Work out the finished part from the listing and answer in its coordinate system (mm). Face numbers are marked on the shaded views. Coordinates: 2 decimals unless noted, no trailing zeros. Loops run counter-clockwise (first coordinate to the right, second up) from the corner with the lowest first, then second, coordinate; pieces in that order, holes last. Notation, with made-up numbers: (21, -17) -> (37, -17) arc R25 cw to (37, -1) -> close; hole circle Ø1 at (74.25, 80.25). An arc over 180 degrees is marked (long way). Use a Markdown table: item, result. Add a question column.
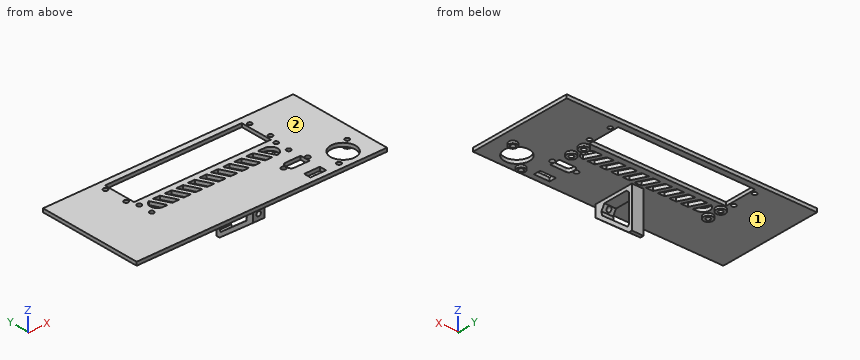
```python
from build123d import *
from OCP.BRepFilletAPI import BRepFilletAPI_MakeChamfer

# Parameters (mm, degrees)
SZKIC1_W                    = 215
SZKIC1_H                    = 90
DODANIE_WYCI_GNI_CIE1_DEPTH = 3
DODANIE_WYCI_GNI_CIE3_DEPTH = 5
SZKIC4_R                    = 1.9
WYTNIJ_WYCI_GNI_CIE1_DEPTH  = 10
SZKIC5_R                    = 1.9
SZKIC5_W                    = 117.5
SZKIC5_H                    = 28
WYTNIJ_WYCI_GNI_CIE2_DEPTH  = 35
SFAZOWANIE1_SIZE            = 2
SFAZOWANIE1_SIZE2           = 1.42483793
SFAZOWANIE1_SIZE2_2         = 2.349845037
SZKIC6_R                    = 10.75
SZKIC6_R_2                  = 1.9
SZKIC6_R_3                  = 2
SZKIC6_W                    = 13.5
SZKIC6_H                    = 6
WYTNIJ_WYCI_GNI_CIE3_DEPTH  = 237.154610372
SZKIC8_R                    = 3.5
SZKIC8_R_2                  = 2
DODANIE_WYCI_GNI_CIE4_DEPTH = 2
SZKIC9_R                    = 1.9
WYTNIJ_WYCI_GNI_CIE4_DEPTH  = 3
DODANIE_WYCI_GNI_CIE5_START = 2
SZKIC10_R                   = 4
SZKIC10_R_2                 = 1.9
DODANIE_WYCI_GNI_CIE5_DEPTH = 2


with BuildPart() as part:
    # Szkic1 → Dodanie-wyciągnięcie1 (new body)
    with BuildSketch(Plane.XY):
        with Locations((107.5, 45)):
            Rectangle(SZKIC1_W, SZKIC1_H)
    extrude(amount=DODANIE_WYCI_GNI_CIE1_DEPTH)

    # Szkic3 → Dodanie-wyciągnięcie3 (add, symmetric)
    with BuildSketch(Plane(origin=(107.5, 0, 0), x_dir=(0, 0, -1), z_dir=(1, 0, 0))):
        Polygon((0, 3), (10, 3), (35, 35), (35, 38), (0, 38), align=None)
        Polygon((3, 11.541451884), (3, 35), (31.193011155, 35), (9.799205499, 7.615928759), align=None, mode=Mode.SUBTRACT)
    extrude(amount=DODANIE_WYCI_GNI_CIE3_DEPTH, both=True)

    # Szkic4 → Wytnij-wyciągnięcie1 (cut)
    with BuildSketch(Plane.XZ.offset(-3)):
        with Locations(Location((107.5, -5, 0), (0, 0, 270))):
            Circle(SZKIC4_R)
    extrude(amount=-WYTNIJ_WYCI_GNI_CIE1_DEPTH, mode=Mode.SUBTRACT)

    # Szkic5 → Wytnij-wyciągnięcie2 (cut)
    with BuildSketch(Plane.XY.offset(3)):
        with Locations((45.5, 81)):
            Circle(SZKIC5_R)
        with Locations((45.5, 61)):
            Circle(SZKIC5_R)
        with Locations((169.5, 61)):
            Circle(SZKIC5_R)
        with Locations((169.5, 81)):
            Circle(SZKIC5_R)
        with Locations((107.5, 71)):
            Rectangle(SZKIC5_W, SZKIC5_H)
    extrude(amount=-WYTNIJ_WYCI_GNI_CIE2_DEPTH, mode=Mode.SUBTRACT)

    # Sfazowanie1: one chamfer whose edges measure the first distance from different faces: ONE call of the kernel's chamfer builder (chamfer() names one face for all edges)
    sfazowanie1_edges_1 = [part.edges().sort_by_distance(p)[0] for p in [
        (107.5, 35, -31.193011155),
    ]]
    sfazowanie1_side_1 = [part.faces().sort_by_distance(p)[0] for p in [
        (107.5, 35, -17.096505578),
    ]]
    sfazowanie1_edges_2 = [part.edges().sort_by_distance(p)[0] for p in [
        (107.5, 35, -3),
    ]]
    sfazowanie1_edges_3 = [part.edges().sort_by_distance(p)[0] for p in [
        (107.5, 7.615928759, -9.799205499),
    ]]
    sfazowanie1_side_3 = [part.faces().sort_by_distance(p)[0] for p in [
        (107.5, 21.30796438, -20.496108327),
    ]]
    sfazowanie1 = BRepFilletAPI_MakeChamfer(part.part.solid().wrapped)
    for e in sfazowanie1_edges_1:
        sfazowanie1.Add(SFAZOWANIE1_SIZE, SFAZOWANIE1_SIZE2, e.wrapped, sfazowanie1_side_1[0].wrapped)  # the first distance lies on this face
    for e in sfazowanie1_edges_2:
        sfazowanie1.Add(SFAZOWANIE1_SIZE, e.wrapped)
    for e in sfazowanie1_edges_3:
        sfazowanie1.Add(SFAZOWANIE1_SIZE, SFAZOWANIE1_SIZE2_2, e.wrapped, sfazowanie1_side_3[0].wrapped)  # the first distance lies on this face
    add(Compound.cast(sfazowanie1.Shape()), mode=Mode.REPLACE)

    # Szkic6 → Wytnij-wyciągnięcie3 (cut, through all)
    with BuildSketch(Plane.XY.offset(3)):
        with Locations((191, 15.35)):
            Circle(SZKIC6_R)
        with Locations((203, 24.85)):
            Circle(SZKIC6_R_2)
        with Locations((179, 5.85)):
            Circle(SZKIC6_R_2)
        with Locations((148.5, 25.05)):
            Circle(SZKIC6_R_3)
        with Locations((169.25, 25.05)):
            Circle(SZKIC6_R_3)
        with Locations((160.25, 7.8)):
            Rectangle(SZKIC6_W, SZKIC6_H)
        with BuildLine():
            Line((167, 20.8), (153.9, 20.8))
            ThreePointArc((153.9, 20.8), (151.849390335, 21.649390335), (151, 23.7))
            Line((151, 23.7), (151, 26.4))
            ThreePointArc((151, 26.4), (151.849390335, 28.450609665), (153.9, 29.3))
            Line((153.9, 29.3), (167, 29.3))
            Line((167, 29.3), (167, 20.8))
        make_face()
    extrude(amount=-WYTNIJ_WYCI_GNI_CIE3_DEPTH, mode=Mode.SUBTRACT)

    # Szkic8 → Dodanie-wyciągnięcie4 (add)
    # profile 1 of 2: a face of its own
    with BuildSketch(Plane(origin=(0, 0, 0), x_dir=(-1, 0, 0), z_dir=(0, 0, -1))):
        with Locations((-179, 5.85)):
            Circle(SZKIC8_R)
        with Locations((-179, 5.85)):
            Circle(SZKIC8_R_2, mode=Mode.SUBTRACT)
    # profile 2 of 2: a face of its own
    with BuildSketch(Plane(origin=(0, 0, 0), x_dir=(-1, 0, 0), z_dir=(0, 0, -1))):
        with Locations((-203, 24.85)):
            Circle(SZKIC8_R)
        with Locations((-203, 24.85)):
            Circle(SZKIC8_R_2, mode=Mode.SUBTRACT)
    extrude(amount=DODANIE_WYCI_GNI_CIE4_DEPTH)

    # Szkic9 → Wytnij-wyciągnięcie4 (cut)
    with BuildSketch(Plane(origin=(0, 0, 0), x_dir=(-1, 0, 0), z_dir=(0, 0, -1))):
        with Locations((-166.25, 52)):
            Circle(SZKIC9_R)
        with Locations((-166.25, 40)):
            Circle(SZKIC9_R)
        with BuildLine():
            Line((-150.385024789, 52), (-156.25, 52))
            ThreePointArc((-156.25, 52), (-162.25, 46), (-156.25, 40))
            Line((-156.25, 40), (-150.385024789, 52))
        make_face()
        Polygon((-140.385024789, 52), (-146.385024789, 52), (-152.25, 40), (-146.25, 40), align=None)
        Polygon((-130.385024789, 52), (-136.385024789, 52), (-142.25, 40), (-136.25, 40), align=None)
        Polygon((-120.385024789, 52), (-126.385024789, 52), (-132.25, 40), (-126.25, 40), align=None)
        Polygon((-110.385024789, 52), (-116.385024789, 52), (-122.25, 40), (-116.25, 40), align=None)
        Polygon((-100.385024789, 52), (-106.385024789, 52), (-112.25, 40), (-106.25, 40), align=None)
        Polygon((-90.385024789, 52), (-96.385024789, 52), (-102.25, 40), (-96.25, 40), align=None)
        Polygon((-80.385024789, 52), (-86.385024789, 52), (-92.25, 40), (-86.25, 40), align=None)
        Polygon((-70.385024789, 52), (-76.385024789, 52), (-82.25, 40), (-76.25, 40), align=None)
        Polygon((-60.385024789, 52), (-66.385024789, 52), (-72.25, 40), (-66.25, 40), align=None)
        with BuildLine():
            Line((-56.582969685, 51.594995944), (-62.25, 40))
            Line((-62.25, 40), (-58.75, 40))
            ThreePointArc((-58.75, 40), (-52.852120056, 44.897724096), (-56.582969685, 51.594995944))
        make_face()
        with Locations((-48.75, 40)):
            Circle(SZKIC9_R)
        with Locations((-48.75, 52)):
            Circle(SZKIC9_R)
    extrude(amount=-WYTNIJ_WYCI_GNI_CIE4_DEPTH, mode=Mode.SUBTRACT)

    # Szkic10 → Dodanie-wyciągnięcie5 (add)
    # profile 1 of 4: a face of its own
    with BuildSketch(Plane(origin=(0, 0, 0), x_dir=(-1, 0, 0), z_dir=(0, 0, -1)).offset(DODANIE_WYCI_GNI_CIE5_START)):
        with Locations((-166.25, 52)):
            Circle(SZKIC10_R)
        with Locations((-166.25, 52)):
            Circle(SZKIC10_R_2, mode=Mode.SUBTRACT)
    # profile 2 of 4: a face of its own
    with BuildSketch(Plane(origin=(0, 0, 0), x_dir=(-1, 0, 0), z_dir=(0, 0, -1)).offset(DODANIE_WYCI_GNI_CIE5_START)):
        with Locations((-166.25, 40)):
            Circle(SZKIC10_R)
        with Locations((-166.25, 40)):
            Circle(SZKIC10_R_2, mode=Mode.SUBTRACT)
    # profile 3 of 4: a face of its own
    with BuildSketch(Plane(origin=(0, 0, 0), x_dir=(-1, 0, 0), z_dir=(0, 0, -1)).offset(DODANIE_WYCI_GNI_CIE5_START)):
        with Locations((-48.75, 40)):
            Circle(SZKIC10_R)
        with Locations((-48.75, 40)):
            Circle(SZKIC10_R_2, mode=Mode.SUBTRACT)
    # profile 4 of 4: a face of its own
    with BuildSketch(Plane(origin=(0, 0, 0), x_dir=(-1, 0, 0), z_dir=(0, 0, -1)).offset(DODANIE_WYCI_GNI_CIE5_START)):
        with Locations((-48.75, 52)):
            Circle(SZKIC10_R)
        with Locations((-48.75, 52)):
            Circle(SZKIC10_R_2, mode=Mode.SUBTRACT)
    extrude(amount=-DODANIE_WYCI_GNI_CIE5_DEPTH)


solid = part.part
```
Item 1: For a pull along X with two mould halves and no side action, classify the marked faces 1 and 2 as +X half, -X half, draft (parallel to the pull), parting line (faces both ways), or undercut.
Item 2: Find the intervals of material crossed by probe 1 along Y at (x, z) = (169.5, 0.5); probe 2 along Y at (x, z) = (191, 2); probe 3 along Y at (x, z) = (45, 1), in increasing order.
Item 3: Section A-A (z = -17.5) is taken. Determine the outline of the cut face in (x, y).
Item 4: Section B-B (y = 46) is taken. Count the separate pieces of the cut face and the enclosed holes in it, then the cut area to 4 significant figures.
Item 5: Given pin 1 (4 mm diameter, centred on x = 167, y = 51, fed in from -Z); pin 2 (11 mm diameter, centred on x = 110, y = 21.5, fed in from -Z), each flat-ended and moving along its own axis, determine where each tip first touches the part or whether it passes through.
Output:
| question | item | result |
|---|---|---|
| 1 | face 1 | undercut |
| 1 | face 2 | draft |
| 2 | probe 1 | y = 0 to 23.07, 27.03 to 59.1, 62.9 to 79.1, 82.9 to 90 |
| 2 | probe 2 | y = 0 to 4.6, 26.1 to 90 |
| 2 | probe 3 | y = 0 to 59.17, 62.83 to 79.17, 82.83 to 90 |
| 3 | outline | (102.5, 12.6) -> (112.5, 12.6) -> (112.5, 17.47) -> (102.5, 17.47) -> close; (102.5, 35) -> (112.5, 35) -> (112.5, 38) -> (102.5, 38) -> close |
| 4 | separate pieces | 12 |
| 4 | enclosed holes | 0 |
| 4 | area | 436.5 mm2 |
| 5 | pin 1 | stops at z = -2 |
| 5 | pin 2 | stops at z = -28.75 |
